Part model, mm, in its own coordinate system. Coordinates: 2 decimals unless noted, no trailing zeros. Loops run counter-clockwise (first coordinate to the right, second up) from the corner with the lowest first, then second, coordinate; pieces in that order, holes last. Notation, with made-up numbers: M 2,77 L 32,77 A19 cw 32,97 Z; hole C 63,-26 d9. An arc over 180 degrees is marked long. Use a Markdown table: item, result. Add a question column.
1) Wall check: probe 1 along X at (y, z) = (15.25, 0); probe 2 along Z at (x, y) = (21, 15.75); probe 3 along X at (y, z) = (21.75, 1.2). Give the ranges that are in metal, low to high. Write a range as from..to.
2) Pin check, flat tip, straight feed: pin 1 Ø1 at (x, z) = (-49.5, 1.5) entering from -Y. Stop position of the tip, or through.
3) Pull direction Z, two halves, no side cores. Call faces 1 (the flat face through (-4, 27, 0)), 2 (the flat face through (-4, 13, 2.5)), 3 (the cylindrical face through (22.276, 13.311, 0.314)): released by +Z, released by -Z, zero draft, split by the parting line, or undercut.
4) Band-saw the part on C-C (y = 12). List the corners of the cut face in (x, z), plus the area to 3 significant figures.
5) Band-saw the part on B-B (z = 0). List the corners of the cut face in (x, y), plus the area to 3 significant figures.
6) Band-saw the part on A-A (x = 20.86). List the corners of the cut face in (y, z), plus the area to 3 significant figures.
from build123d import *

# Parameters (mm, degrees)
SKETCH_1_W          = 117
SKETCH_1_H          = 5
EXTRUDE_1_DEPTH     = 27
SKETCH_2_R          = 1.45
CUT_EXTRUDE_1_DEPTH = 30


with BuildPart() as part:
    # 草图1 → 凸台-拉伸1 (new body)
    with BuildSketch(Plane(origin=(0, 0, 0), x_dir=(1, 0, 0), z_dir=(0, 1, 0))):
        with Locations((-3.5, 0)):
            Rectangle(SKETCH_1_W, SKETCH_1_H)
    extrude(amount=EXTRUDE_1_DEPTH)

    # 草图2 → 切除-拉伸1 (cut)
    with BuildSketch(Plane(origin=(0, 0, 0), x_dir=(1, 0, 0), z_dir=(0, 1, 0))):
        with Locations(Location((-20.86, 0, 0), (0, 0, 270))):
            Circle(SKETCH_2_R)
        with Locations(Location((20.86, 0, 0), (0, 0, 90))):
            Circle(SKETCH_2_R)
    extrude(amount=CUT_EXTRUDE_1_DEPTH, mode=Mode.SUBTRACT)


solid = part.part
Entries:
| question | item | result |
|---|---|---|
| 1 | probe 1 | -62..-22.31, -19.41..19.41, 22.31..55 |
| 1 | probe 2 | -2.5..-1.44, 1.44..2.5 |
| 1 | probe 3 | -62..-21.67, -20.05..20.05, 21.67..55 |
| 2 | pin 1 | y = 0 |
| 3 | face 1 | zero draft |
| 3 | face 2 | released by +Z |
| 3 | face 3 | undercut |
| 4 | outline | M -62,-2.5 L 55,-2.5 L 55,2.5 L -62,2.5 Z; hole C -20.86,0 d2.9; hole C 20.86,0 d2.9 |
| 4 | area | 572 mm2 |
| 5 | outline | M -62,0 L -22.31,0 L -22.31,27 L -62,27 Z; M -19.41,0 L 19.41,0 L 19.41,27 L -19.41,27 Z; M 22.31,0 L 55,0 L 55,27 L 22.31,27 Z |
| 5 | area | 3,000 mm2 |
| 6 | outline | M 0,-2.5 L 27,-2.5 L 27,-1.45 L 0,-1.45 Z; M 0,1.45 L 27,1.45 L 27,2.5 L 0,2.5 Z |
| 6 | area | 56.7 mm2 |
